Read the model definition and answer for the solid it produces. Units are mm, in the model's axes. Coordinates: 2 decimals unless noted, no trailing zeros. Loops run counter-clockwise (first coordinate to the right, second up) from the corner with the lowest first, then second, coordinate; pieces in that order, holes last. Notation, with made-up numbers: (73, 83.25) - (129, 83.25) arc R21 cw to (129, 112.25) - close; hole circle Ø11 at (-18.75, 50). An arc over 180 degrees is marked (long way). One line per question, with ' | ' between items. Start each with the question number.
```python
from build123d import *

# Parameters (mm, degrees)
F0_W     = 350
F0_H     = 20
F1_DEPTH = 20
F3_D     = 9
F5_D     = 9
F7_D     = 9
F8_W     = 100
F8_H     = 20
F8_R     = 4.5
F9_DEPTH = 25


with BuildPart() as f1:
    # F0 (on Top) → F1 (new body)
    with BuildSketch(Plane.XY):
        with Locations((63.1421148777, 26.3889993745)):
            Rectangle(F0_W, F0_H)
    extrude(amount=F1_DEPTH)

    # F3 (through all)
    with Locations(Plane.XY.offset(20)):
        with Locations((-43.5278851223, 26.3889993745), (49.8121148777, 26.3889993745)):
            Hole(F3_D / 2)

    # F5 (through all)
    with Locations(Plane.XY.offset(20)):
        with Locations((-101.8578851223, 26.3889993745), (228.1421148777, 26.3889993745)):
            Hole(F5_D / 2)

    # F7 (through all)
    with Locations(Plane.XY.offset(20)):
        with Locations((16.4721148777, 26.3889993745), (109.8121148777, 26.3889993745)):
            Hole(F7_D / 2)

    # F8 (on face) → F9 (cut)
    with BuildSketch(Plane.XY.offset(20)):
        with Locations((188.1421148777, 26.3889993745)):
            Rectangle(F8_W, F8_H)
        with Locations((228.1421148777, 26.3889993745)):
            Circle(F8_R, mode=Mode.SUBTRACT)
    extrude(amount=-F9_DEPTH, mode=Mode.SUBTRACT)


solid = f1.part
```
1) The part is cut by section B-B on z = 5.5. Write down the section's boundary in (x, y), and give its area (3 significant figures).
2) The part is cut by section D-D on x = 47.5. Write down the section's boundary in (y, z).
3) The mould has two halves that part along Y. Classify faces 1 (the flat face through (11, 36.389, 10)), 2 (the flat face through (11, 27, 20)), 3 (the cylindrical face through (-101.27, 30.85, 9.86)): released by +Y, released by -Y, zero draft, split by the parting line, or undercut.
4) Given pin 1 Ø7 at (x, y) = (16.47, 26.39) entering from +Z, flat-ended and moving along its own axis, determine where the tip first touches the part or whether it passes through.
5) The part is cut by section C-C on y = 24. Write down the section's boundary in (x, z), and give its area (3 significant figures).
6) The part is cut by section A-A on x = -44. Write down the section's boundary in (y, z).
7) Find the intervals of material crossed by line 1 along X through (y, z) = (23, 14.75); line 2 along X through (y, z) = (22.5, 18); line 3 along Y through (x, z) = (17, 3.5), in increasing order. Write a range as from..to.
Answer below:
1) outline: (-111.86, 16.39) - (138.14, 16.39) - (138.14, 36.39) - (-111.86, 36.39) - close; hole circle Ø9 at (-101.86, 26.39); hole circle Ø9 at (-43.53, 26.39); hole circle Ø9 at (16.47, 26.39); hole circle Ø9 at (49.81, 26.39); hole circle Ø9 at (109.81, 26.39) | area: 4,680 mm2
2) outline: (16.39, 0) - (22.53, 0) - (22.53, 20) - (16.39, 20) - close; (30.25, 0) - (36.39, 0) - (36.39, 20) - (30.25, 20) - close
3) face 1: released by +Y | face 2: zero draft | face 3: undercut
4) pin 1: through
5) outline: (-111.86, 0) - (-105.67, 0) - (-105.67, 20) - (-111.86, 20) - close; (-98.04, 0) - (-47.34, 0) - (-47.34, 20) - (-98.04, 20) - close; (-39.71, 0) - (12.66, 0) - (12.66, 20) - (-39.71, 20) - close; (20.29, 0) - (46, 0) - (46, 20) - (20.29, 20) - close; (53.63, 0) - (106, 0) - (106, 20) - (53.63, 20) - close; (113.63, 0) - (138.14, 0) - (138.14, 20) - (113.63, 20) - close | area: 4,240 mm2
6) outline: (16.39, 0) - (21.91, 0) - (21.91, 20) - (16.39, 20) - close; (30.86, 0) - (36.39, 0) - (36.39, 20) - (30.86, 20) - close
7) line 1: -111.86..-104.82, -98.9..-46.49, -40.57..13.51, 19.43..46.85, 52.77..106.85, 112.77..138.14 | line 2: -111.86..-104.12, -99.59..-45.79, -41.26..14.21, 18.74..47.55, 52.08..107.55, 112.08..138.14 | line 3: 16.39..21.92, 30.86..36.39
